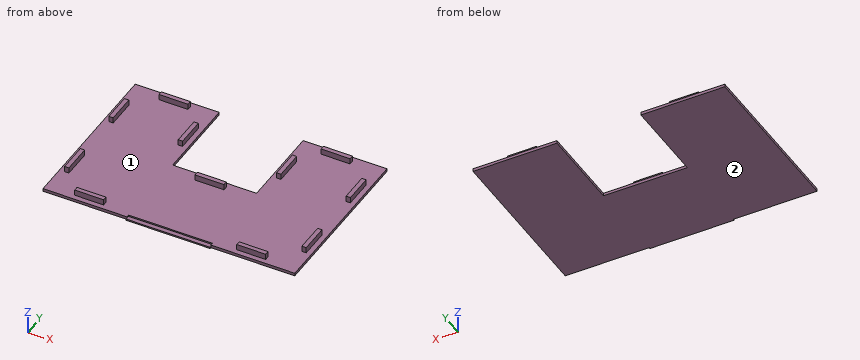
```python
from build123d import *

# Parameters (mm, degrees)
BOX013_W     = 20
BOX013_H     = 3
BOX013_DEPTH = 6
BOX012_W     = 20
BOX012_H     = 3
BOX012_DEPTH = 6
BOX011_W     = 20
BOX011_H     = 3
BOX011_DEPTH = 6
BOX010_W     = 20
BOX010_H     = 3
BOX010_DEPTH = 6
BOX009_W     = 20
BOX009_H     = 3
BOX009_DEPTH = 6
BOX008_W     = 20
BOX008_H     = 3
BOX008_DEPTH = 6
BOX007_W     = 20
BOX007_H     = 3
BOX007_DEPTH = 6
BOX006_W     = 20
BOX006_H     = 3
BOX006_DEPTH = 6
BOX005_W     = 20
BOX005_H     = 3
BOX005_DEPTH = 6
BOX004_W     = 20
BOX004_H     = 3
BOX004_DEPTH = 6
BOX003_W     = 20
BOX003_H     = 3
BOX003_DEPTH = 6
BOX002_W     = 58
BOX002_H     = 117
BOX002_DEPTH = 2
BOX001_W     = 58
BOX001_H     = 117
BOX001_DEPTH = 2
BOX_W        = 58
BOX_H        = 56
BOX_DEPTH    = 2
BOX014_W     = 58
BOX014_H     = 3
BOX014_DEPTH = 1


with BuildPart() as cube013:
    # Box013 → Box013 (new body)
    with BuildSketch(Plane(origin=(77, 51.5, 0), x_dir=(1, 0, 0), z_dir=(0, 0, 1))):
        with Locations((10, 1.5)):
            Rectangle(BOX013_W, BOX013_H)
    extrude(amount=BOX013_DEPTH)


with BuildPart() as cube012:
    # Box012 → Box012 (new body)
    with BuildSketch(Plane(origin=(3.5, 41, 0), x_dir=(0, -1, 0), z_dir=(0, 0, 1))):
        with Locations((10, 1.5)):
            Rectangle(BOX012_W, BOX012_H)
    extrude(amount=BOX012_DEPTH)


with BuildPart() as cube011:
    # Box011 → Box011 (new body)
    with BuildSketch(Plane(origin=(3.5, 97, 0), x_dir=(0, -1, 0), z_dir=(0, 0, 1))):
        with Locations((10, 1.5)):
            Rectangle(BOX011_W, BOX011_H)
    extrude(amount=BOX011_DEPTH)


with BuildPart() as cube010:
    # Box010 → Box010 (new body)
    with BuildSketch(Plane(origin=(51.5, 97, 0), x_dir=(0, -1, 0), z_dir=(0, 0, 1))):
        with Locations((10, 1.5)):
            Rectangle(BOX010_W, BOX010_H)
    extrude(amount=BOX010_DEPTH)


with BuildPart() as cube009:
    # Box009 → Box009 (new body)
    with BuildSketch(Plane(origin=(167.5, 97, 0), x_dir=(0, -1, 0), z_dir=(0, 0, 1))):
        with Locations((10, 1.5)):
            Rectangle(BOX009_W, BOX009_H)
    extrude(amount=BOX009_DEPTH)


with BuildPart() as cube008:
    # Box008 → Box008 (new body)
    with BuildSketch(Plane(origin=(167.5, 41, 0), x_dir=(0, -1, 0), z_dir=(0, 0, 1))):
        with Locations((10, 1.5)):
            Rectangle(BOX008_W, BOX008_H)
    extrude(amount=BOX008_DEPTH)


with BuildPart() as cube007:
    # Box007 → Box007 (new body)
    with BuildSketch(Plane(origin=(119.5, 97, 0), x_dir=(0, -1, 0), z_dir=(0, 0, 1))):
        with Locations((10, 1.5)):
            Rectangle(BOX007_W, BOX007_H)
    extrude(amount=BOX007_DEPTH)


with BuildPart() as cube006:
    # Box006 → Box006 (new body)
    with BuildSketch(Plane(origin=(132, 110.5, 0), x_dir=(1, 0, 0), z_dir=(0, 0, 1))):
        with Locations((10, 1.5)):
            Rectangle(BOX006_W, BOX006_H)
    extrude(amount=BOX006_DEPTH)


with BuildPart() as cube005:
    # Box005 → Box005 (new body)
    with BuildSketch(Plane(origin=(132, 3.5, 0), x_dir=(1, 0, 0), z_dir=(0, 0, 1))):
        with Locations((10, 1.5)):
            Rectangle(BOX005_W, BOX005_H)
    extrude(amount=BOX005_DEPTH)


with BuildPart() as cube004:
    # Box004 → Box004 (new body)
    with BuildSketch(Plane(origin=(20, 3.5, 0), x_dir=(1, 0, 0), z_dir=(0, 0, 1))):
        with Locations((10, 1.5)):
            Rectangle(BOX004_W, BOX004_H)
    extrude(amount=BOX004_DEPTH)


with BuildPart() as cube003:
    # Box003 → Box003 (new body)
    with BuildSketch(Plane(origin=(20, 110.5, 0), x_dir=(1, 0, 0), z_dir=(0, 0, 1))):
        with Locations((10, 1.5)):
            Rectangle(BOX003_W, BOX003_H)
    extrude(amount=BOX003_DEPTH)


with BuildPart() as cube002:
    # Box002 → Box002 (new body)
    with BuildSketch(Plane(origin=(116, 0, 0), x_dir=(1, 0, 0), z_dir=(0, 0, 1))):
        with Locations((29, 58.5)):
            Rectangle(BOX002_W, BOX002_H)
    extrude(amount=BOX002_DEPTH)


with BuildPart() as cube001:
    # Box001 → Box001 (new body)
    with BuildSketch(Plane.XY):
        with Locations((29, 58.5)):
            Rectangle(BOX001_W, BOX001_H)
    extrude(amount=BOX001_DEPTH)


with BuildPart() as cube:
    # Box → Box (new body)
    with BuildSketch(Plane(origin=(58, 2, 0), x_dir=(1, 0, 0), z_dir=(0, 0, 1))):
        with Locations((29, 28)):
            Rectangle(BOX_W, BOX_H)
    extrude(amount=BOX_DEPTH)


with BuildPart() as fusion:
    # Box014 → Box014 (new body)
    with BuildSketch(Plane(origin=(58, -1, 0), x_dir=(1, 0, 0), z_dir=(0, 0, 1))):
        with Locations((29, 1.5)):
            Rectangle(BOX014_W, BOX014_H)
    extrude(amount=BOX014_DEPTH)

    # Fusion: union Cube013, Cube012, Cube011, Cube010, Cube009, Cube008, Cube007, Cube006, Cube005, Cube004, Cube003, Cube002, Cube001, Cube
    add(cube013.part)
    add(cube012.part)
    add(cube011.part)
    add(cube010.part)
    add(cube009.part)
    add(cube008.part)
    add(cube007.part)
    add(cube006.part)
    add(cube005.part)
    add(cube004.part)
    add(cube003.part)
    add(cube002.part)
    add(cube001.part)
    add(cube.part)


solid = fusion.part
```
Input: part model. Units: mm. Frame: model coordinates. Face numbers are marked on the shaded views. Give positions to 0.01 mm unless a question says otherwise; leave off trailing zeros. Order: outer loops, then holes, each group sorted by start corner. A loop starts at its lowest first (then second) coordinate and runs counter-clockwise, first axis right, second up.
1. Cut plane D-D (y = 24.5). Return loops of the section in (x, z).
Computed:
outline: (0, 0) - (174, 0) - (174, 2) - (170.5, 2) - (170.5, 6) - (167.5, 6) - (167.5, 2) - (6.5, 2) - (6.5, 6) - (3.5, 6) - (3.5, 2) - (0, 2) - close
2. Line query: probe 1 along X at (y, z) = (79, 5.6); probe 2 along X at (y, z) = (25, 3.85); probe 3 along X at (y, z) = (69.5, 1.55). Output: solid intervals per line, ascending.
Computed:
probe 1: x = 3.5 to 6.5, 51.5 to 54.5, 119.5 to 122.5, 167.5 to 170.5
probe 2: x = 3.5 to 6.5, 167.5 to 170.5
probe 3: x = 0 to 58, 116 to 174
3. Cut plane C-C (z = 3.9). State how many separate pieces and enclosed holes the cut face has, and give its area (3 significant figures).
Computed:
separate pieces: 11
enclosed holes: 0
area: 660 mm2
4. Cut plane A-A (y = 61.5). Return loops of the section in (x, z).
Computed:
outline: (0, 0) - (58, 0) - (58, 2) - (0, 2) - close; (116, 0) - (174, 0) - (174, 2) - (116, 2) - close
5. Cut plane B-B (x = 93.5). Return loops of the section in (y, z).
Computed:
outline: (-1, 0) - (58, 0) - (58, 2) - (54.5, 2) - (54.5, 6) - (51.5, 6) - (51.5, 2) - (2, 2) - (2, 1) - (-1, 1) - close
6. Draft query along Y for the marked faces 1 and 2. Return one class per face: released by +Y, released by -Y, zero draft, split by the parting line, or undercut.
Computed:
face 1: undercut
face 2: zero draft
7. Pin query (flat end, axial travel): pin 1 Ø1.5 at (y, z) = (5.5, 3.5) entering from +X; pin 2 Ø2 at (x, z) = (141, 4) entering from +Y; pin 3 Ø3 at (y, z) = (41, 5) entering from +X. Return the tip coordinate at first contact, or that it passes through.
Computed:
pin 1: stops at x = 152
pin 2: stops at y = 113.5
pin 3: stops at x = 170.5
